Check sheet for the modelled part. Datum: model origin and axes. Units: mm. Give positions to 0.01 mm unless a question says otherwise; leave off trailing zeros. Loops run counter-clockwise (first coordinate to the right, second up) from the corner with the lowest first, then second, coordinate; pieces in that order, holes last. Notation, with made-up numbers: (-10.5, 22.5) -> (48.5, 22.5) arc R8 cw to (48.5, 30.5) -> close; hole circle Ø9 at (84, 25). An arc over 180 degrees is marked (long way). Answer as CSV lines item,"result". Start each with the question number.
(1) Release check for a two-part mould opening along Y. For faces 1 (the face through (-80.867, -71.905, 0.507)), 2 (the face through (147.58, 2.41, 0.49)), 3 (the face through (12, 16, 0)) record: pulls with the +Y half, pulls with the -Y half, needs draft (parallel to the pull), parting line crosses it, or undercut.
(2) Gauge pin test, flat end, axial feed: pin 1 Ø1 at (x, y) = (-41.5, 16) entering from -Z. Record the tip position at first contact, or that the pin passes through.
(3) Section check C-C on y = 25.5. Enter the section's corners in (x, z), plus the area to 3 significant figures.
(4) Section check B-B on y = -43.5. Enter the section's corners in (x, z).
(5) Section check A-A on z = 0.3. State how many separate pieces and enclosed holes the cut face has, plus the area to 3 significant figures.
(6) Material ranges on line 1 (X direction, y = 94.5, z = 0.55); line 2 (Y direction, x = -67, z = 0.5); line 3 (Y direction, x = 54.5, z = 0.65), recorded low to high. Write a range as from..to.
from build123d import *

# Parameters (mm, degrees)
SKETCH1_W           = 200
SKETCH1_H           = 160
SKETCH1_W_2         = 292.37604307
SKETCH1_H_2         = 30
BOSS_EXTRUDE1_DEPTH = 1
FILLET1_R           = 10
SKETCH2_R           = 4
SKETCH2_R_2         = 11
SKETCH2_R_3         = 1.5
CUT_EXTRUDE1_DEPTH  = 3


with BuildPart() as part:
    # Sketch1 → Boss-Extrude1 (new body)
    with BuildSketch(Plane.XY):
        Rectangle(SKETCH1_W, SKETCH1_H)
        Polygon((192.37604307, 80), (100, -80), (100, 80), align=None)
        with Locations((46.188021535, 95)):
            Rectangle(SKETCH1_W_2, SKETCH1_H_2)
    extrude(amount=BOSS_EXTRUDE1_DEPTH)

    # Fillet1
    fillet1_edges = [part.edges().sort_by_distance(p)[0] for p in [
        (-100, 110, 0.5),
        (192.37604307, 110, 0.5),
        (-100, -80, 0.5),
        (192.37604307, 80, 0.5),
        (100, -80, 0.5),
    ]]
    fillet(fillet1_edges, radius=FILLET1_R)

    # Sketch2 → Cut-Extrude1 (cut)
    with BuildSketch(Plane.XY.offset(1)):
        with Locations((93.07179677, -68)):
            Circle(SKETCH2_R)
        with Locations((177.364936071, 78)):
            Circle(SKETCH2_R)
        with Locations((-67, -10)):
            Circle(SKETCH2_R_2)
        with Locations((-80, -68)):
            Circle(SKETCH2_R)
        with Locations((-53, -10)):
            Circle(SKETCH2_R_3)
        with Locations((-67, 4)):
            Circle(SKETCH2_R_3)
        with Locations((-81, -10)):
            Circle(SKETCH2_R_3)
        with Locations((-67, -24)):
            Circle(SKETCH2_R_3)
        with Locations((35.957265033, 70)):
            Circle(SKETCH2_R)
        with Locations((62.79605759, -67.242640687)):
            Circle(SKETCH2_R_3)
        with Locations((54.310776216, -58.757359313)):
            Circle(SKETCH2_R_3)
        with Locations((-33.274226936, -67.242640687)):
            Circle(SKETCH2_R_3)
        with Locations((-41.75950831, -58.757359313)):
            Circle(SKETCH2_R_3)
        with Locations((14.225855729, -60.5)):
            Circle(SKETCH2_R_3)
        with Locations((-37.754710439, 87.757359313)):
            Circle(SKETCH2_R_3)
        with Locations((-46.239991813, 96.242640687)):
            Circle(SKETCH2_R_3)
        with Locations((-90.295627115, 94.5)):
            Circle(SKETCH2_R_3)
        with BuildLine():
            Line((-79.516586773, 82), (-62.300333374, 82))
            ThreePointArc((-62.300333374, 82), (-58.300333374, 78), (-62.300333374, 74))
            Line((-62.300333374, 74), (-79.516586773, 74))
            ThreePointArc((-79.516586773, 74), (-83.516586773, 78), (-79.516586773, 82))
        make_face()
    extrude(amount=-CUT_EXTRUDE1_DEPTH, mode=Mode.SUBTRACT)


solid = part.part
Working result:
1,face 1,"undercut"
1,face 2,"pulls with the -Y half"
1,face 3,"needs draft"
2,pin 1,"stops at z = 0"
3,outline,"(-100, 0) -> (160.91, 0) -> (160.91, 1) -> (-100, 1) -> close"
3,area,"261 mm^2"
4,outline,"(-100, 0) -> (121.07, 0) -> (121.07, 1) -> (-100, 1) -> close"
5,separate pieces,"1"
5,enclosed holes,"18"
5,area,"47,200 mm^2"
6,line 1,"x = -100..-91.8, -88.8..192.38"
6,line 2,"y = -80..-25.5, -22.5..-21, 1..2.5, 5.5..74, 82..110"
6,line 3,"y = -80..-60.25, -57.27..110"
